Verification items for the finished model (mm, model axes). A direction names the side the tool comes from. Give positions to 0.01 mm unless a question says otherwise; leave off trailing zeros. Write each loop counter-clockwise with the first axis right and the second up, starting at its lowest first coordinate (ties: lowest second). Pieces come first, ordered by that corner, then holes. Notation, with made-up numbers: M -34.75,5.5 L 11.25,5.5 A17 ccw 11.25,37.5 Z; hole C -5,-12 d9. An arc over 180 degrees is marked long. Answer as a JSON object with one key per item and string values.
```python
from build123d import *

# Parameters (mm, degrees)
F0_W     = 914.4
F0_H     = 635
F1_DEPTH = 6.35
F2_DEPTH = 12.7
F3_W     = 127
F3_H     = 381
F4_DEPTH = 73.66


with BuildPart() as f1:
    # F0 (on Top) → F1 (new body, symmetric)
    with BuildSketch(Plane.XY):
        Rectangle(F0_W, F0_H)
    extrude(amount=F1_DEPTH, both=True)

    # F0 (on Top) → F2 (join)
    with BuildSketch(Plane.XY):
        Rectangle(F0_W, F0_H)
    extrude(amount=F2_DEPTH)

    # F3 (on face) → F4 (cut)
    with BuildSketch(Plane(origin=(0, 0, -6.35), x_dir=(1, 0, 0), z_dir=(0, 0, -1))):
        with Locations((-266.7, 0)):
            Rectangle(F3_W, F3_H)
        with Locations((266.7, 0)):
            Rectangle(F3_W, F3_H)
    extrude(amount=-F4_DEPTH, mode=Mode.SUBTRACT)


solid = f1.part
```
1) Section check B-B on x = -267. Record the boundary of the cut face in (y, z), and give its area (3 significant figures).
Completed:
{"outline": "M -317.5,-6.35 L -190.5,-6.35 L -190.5,12.7 L -317.5,12.7 Z; M 190.5,-6.35 L 317.5,-6.35 L 317.5,12.7 L 190.5,12.7 Z", "area": "4,840 mm2"}
2) Thickness scan on L1, parallel to X at y = -59, z = 3.75; L2, parallel to Y at x = -330, z = 4.75. Record the ranges inside material, lowest first.
Completed:
{"L1": "x = -457.2 to -330.2, -203.2 to 203.2, 330.2 to 457.2", "L2": "y = -317.5 to -190.5, 190.5 to 317.5"}
3) Access from +Z, -Z, +X, -X, +Y, -Y to the whole of each face (thin tool, end or side, straight path). Record for faces 1 (the face through (-268, -190.5, 3)), 2 (the face through (-457.2, -4, 3)).
Completed:
{"face 1": "+Z, -Z", "face 2": "+Z, -Z, -X, +Y, -Y"}
4) Section check A-A on z = 9.75. Record the boundary of the cut face in (x, y).
Completed:
{"outline": "M -457.2,-317.5 L 457.2,-317.5 L 457.2,317.5 L -457.2,317.5 Z; hole M -330.2,-190.5 L -203.2,-190.5 L -203.2,190.5 L -330.2,190.5 Z; hole M 203.2,-190.5 L 330.2,-190.5 L 330.2,190.5 L 203.2,190.5 Z"}
5) Section check C-C on y = -181.5. Record the boundary of the cut face in (x, z), and give its area (3 significant figures).
Completed:
{"outline": "M -457.2,-6.35 L -330.2,-6.35 L -330.2,12.7 L -457.2,12.7 Z; M -203.2,-6.35 L 203.2,-6.35 L 203.2,12.7 L -203.2,12.7 Z; M 330.2,-6.35 L 457.2,-6.35 L 457.2,12.7 L 330.2,12.7 Z", "area": "12,600 mm2"}
6) Release check for a two-part mould opening along X. For faces 3 (the face through (266, -190.5, 3)), 4 (the face through (-6, 4, 12.7)), 5 (the face through (457.2, -4, 3)), 6 (the face through (-268, 190.5, 3)) record: pulls with the +X half, pulls with the -X half, needs draft (parallel to the pull), parting line crosses it, or undercut.
Completed:
{"face 3": "undercut", "face 4": "needs draft", "face 5": "pulls with the +X half", "face 6": "undercut"}
